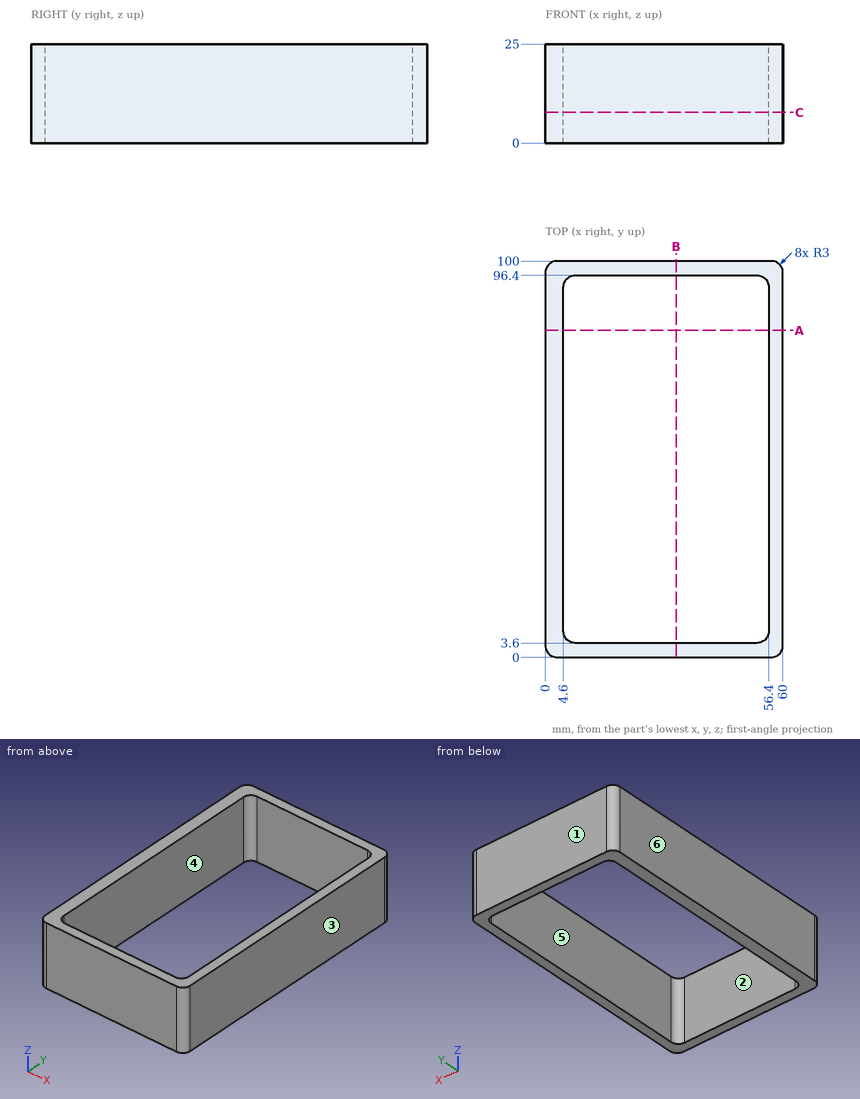
Source: three-view drawing plus pictorial views. Frame: mm from the lowest corner of the part. A direction names the side the tool comes from. Give positions to 0.01 mm unless a question says otherwise; leave off trailing zeros. Order: outer loops, then holes, each group sorted by start corner. A loop starts at its lowest first (then second) coordinate and runs counter-clockwise, first axis right, second up. Notation, with made-up numbers: M 70,-13.5 L 81,-13.5 A36 cw 81,22.5 Z; hole C 77.5,-5 d3. An arc over 180 degrees is marked long. Return JSON: item names as keys, results as strings.
Item 1: Ray query, probe 1 along X at (y, z) = (82, 22.5); probe 2 along Y at (x, z) = (53, 18); probe 3 along Y at (x, z) = (6, 13.75). Return the intervals inside material, ascending.
Solutions:
{"probe 1": "0 to 4.6, 56.4 to 60", "probe 2": "0 to 3.6, 96.4 to 100", "probe 3": "0 to 4.06, 95.94 to 100"}
Item 2: Pull-direction query (X, two-part tool) for the marked faces 1, 2, 3 and 4; classes: +X half, -X half, draft (parallel to the pull), parting line (faces both ways), or undercut.
Solutions:
{"face 1": "draft", "face 2": "undercut", "face 3": "+X half", "face 4": "undercut"}
Item 3: Access query for the marked faces 5 and 6. Directions: +Z, -Z, +X, -X, +Y, -Y. A direction counts if a zero-diameter tool reaches every point of the face in a straight line with its end or side. Return the directions, or none.
Solutions:
{"face 5": "+Z, -Z", "face 6": "+Z, -Z, -X, +Y, -Y"}
Item 4: Cut plane A-A (y = 82.5). Return loops of the section in (x, z).
Solutions:
{"outline": "M 0,0 L 4.6,0 L 4.6,25 L 0,25 Z; M 56.4,0 L 60,0 L 60,25 L 56.4,25 Z"}
Item 5: Cut plane C-C (z = 7.75). Return loops of the section in (x, y).
Solutions:
{"outline": "M 0,3 A3 ccw 3,0 L 57,0 A3 ccw 60,3 L 60,97 A3 ccw 57,100 L 3,100 A3 ccw 0,97 Z; hole M 4.6,6.6 A3 ccw 7.6,3.6 L 53.4,3.6 A3 ccw 56.4,6.6 L 56.4,93.4 A3 ccw 53.4,96.4 L 7.6,96.4 A3 ccw 4.6,93.4 Z"}
Item 6: Cut plane B-B (x = 33). Return loops of the section in (y, z).
Solutions:
{"outline": "M 0,0 L 3.6,0 L 3.6,25 L 0,25 Z; M 96.4,0 L 100,0 L 100,25 L 96.4,25 Z"}
